Drawing for the job (mm, zero at the part's lowest x, y, z). A direction names the side the tool comes from. Coordinates: 2 decimals unless noted, no trailing zeros. Loops run counter-clockwise (first coordinate to the right, second up) from the corner with the lowest first, then second, coordinate; pieces in that order, holes last. Notation, with made-up numbers: (-21.75, 47) - (37.25, 47) arc R31 ccw to (37.25, 84) - close; hole circle Ø5 at (31.5, 52.5). An arc over 180 degrees is marked (long way). One line per item, written item: value.
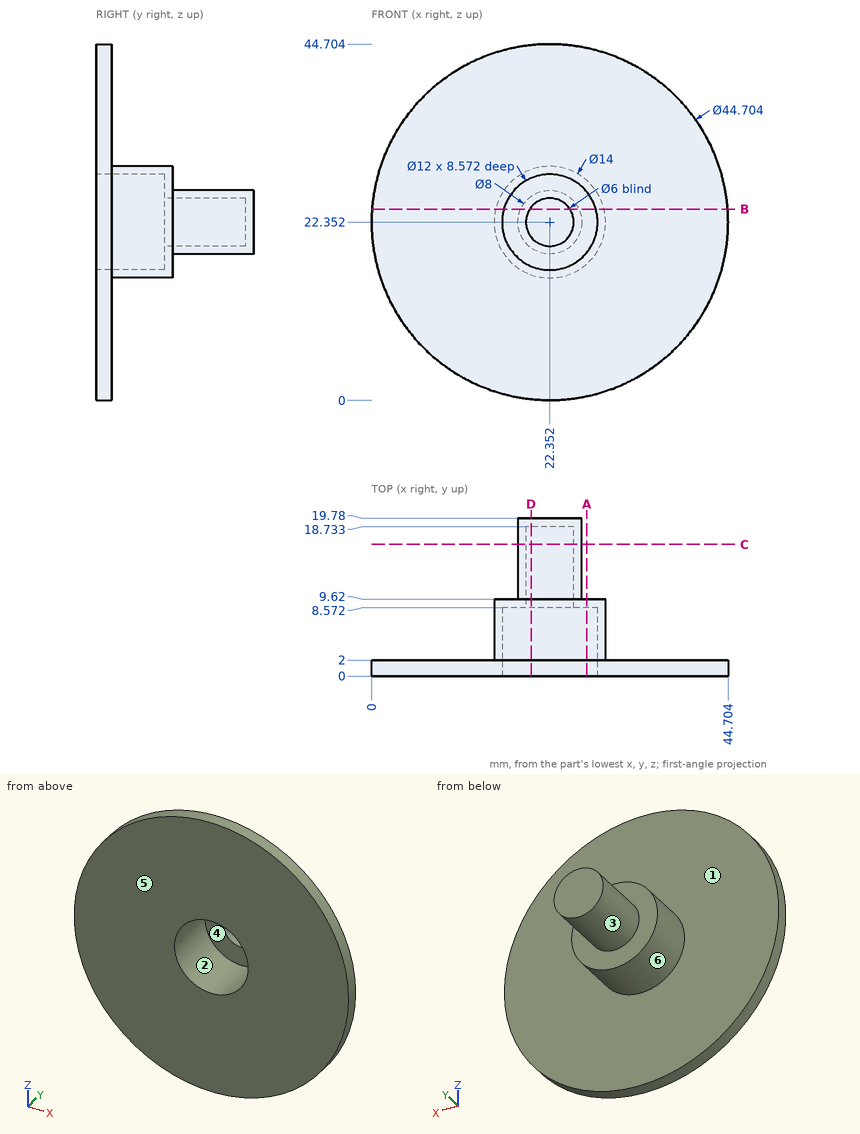
Item 1: Probe probe 1 along Y at (x, z) = (37, 20.5); probe 2 along Y at (x, z) = (22.5, 26.5); probe 3 along X at (y, z) = (6, 19.5) (1 decimal). List the from-to ranges inside material, lowest first. Write a range as from..to.
Check result:
probe 1: y = 0..2
probe 2: y = 8.57..9.62
probe 3: x = 16..17.1, 27.6..28.7
Item 2: Cut at B-B, the plane z = 24. Write the cut outline in (x, y) (1 decimal).
Check result:
outline: (0.1, 0) - (16.6, 0) - (16.6, 8.6) - (19.8, 8.6) - (19.8, 18.7) - (24.9, 18.7) - (24.9, 8.6) - (28.1, 8.6) - (28.1, 0) - (44.6, 0) - (44.6, 2) - (29.2, 2) - (29.2, 9.6) - (26, 9.6) - (26, 19.8) - (18.7, 19.8) - (18.7, 9.6) - (15.5, 9.6) - (15.5, 2) - (0.1, 2) - close
Item 3: Pull direction Z, two halves, no side cores. Call the marked faces 1, 2, 3 and 4: released by +Z, released by -Z, zero draft, split by the parting line, or undercut.
Check result:
face 1: zero draft
face 2: undercut
face 3: split by the parting line
face 4: undercut
Item 4: Tool access for the marked faces 5 and 6: list every direction of +Z, -Z, +X, -X, +Y, -Y with a clear straight run to the whole face (end or side of a thin tool).
Check result:
face 5: +Z, -Z, +X, -X, -Y
face 6: +Y
Item 5: Drop flat-ended pins along their axis: P1, Ø3.5, axis at x = 22, z = 24.5, coming from the -Y side; P2, Ø13.5, axis at x = 30.5, z = 12.5, coming from the +Y side; P3, Ø1.5, axis at x = 22, y = 9.5, coming from the +Z side; P4, Ø6, axis at x = 8, y = 7, coming from the -Z side. Give the stop position or say it passes through.
Check result:
P1: stops at y = 8.57
P2: stops at y = 9.62
P3: stops at z = 29.35
P4: passes through
Item 6: Cut at A-A, the plane x = 27. Write the cut outline in (y, z) (1 decimal), then the cut area to 3 significant figures.
Check result:
outline: (0, 0.5) - (2, 0.5) - (2, 17.1) - (9.6, 17.1) - (9.6, 27.6) - (2, 27.6) - (2, 44.2) - (0, 44.2) - (0, 26.1) - (8.6, 26.1) - (8.6, 18.6) - (0, 18.6) - close
area: 102 mm^2
Item 7: Cut at C-C, the plane y = 16.5. Write the cut outline in (x, z).
Check result:
outline: circle Ø8 at (22.35, 22.35); hole circle Ø6 at (22.35, 22.35)
Item 8: Cut at D-D, the plane x = 20. Write the cut outline in (y, z) (1 decimal).
Check result:
outline: (0, 0.1) - (2, 0.1) - (2, 15.8) - (9.6, 15.8) - (9.6, 19.1) - (19.8, 19.1) - (19.8, 25.6) - (9.6, 25.6) - (9.6, 28.9) - (2, 28.9) - (2, 44.6) - (0, 44.6) - (0, 27.9) - (8.6, 27.9) - (8.6, 24.2) - (18.7, 24.2) - (18.7, 20.5) - (8.6, 20.5) - (8.6, 16.8) - (0, 16.8) - close
